```python
from build123d import *

# Parameters (mm, degrees)
SKETCH1_R               = 6.985
BOSS_EXTRUDE1_DEPTH     = 2.54
BOSS_EXTRUDE2_DEPTH     = 81.28
BOSS_EXTRUDE3_DEPTH     = 2.54
FILLET1_R               = 2.54
SKETCH4_R               = 7.62
BOSS_EXTRUDE4_DEPTH     = 12.7
CUT_EXTRUDE1_DEPTH      = 101.243554531
CUT_EXTRUDE1_DEPTH_BACK = 101.243554531
SKETCH5_R               = 1.905


with BuildPart() as part:
    # Sketch1 → Boss-Extrude1 (new body)
    with BuildSketch(Plane.XY):
        Circle(SKETCH1_R)
    extrude(amount=BOSS_EXTRUDE1_DEPTH)

    # Sketch2 → Boss-Extrude2 (add)
    with BuildSketch(Plane.XY.offset(2.54)):
        Polygon((-0.635, -0.635), (-5.715, -0.635), (-5.715, 0.635), (-0.635, 0.635), (-0.635, 5.715), (0.635, 5.715), (0.635, 0.635), (5.715, 0.635), (5.715, -0.635), (0.635, -0.635), (0.635, -5.715), (-0.635, -5.715), align=None)
    extrude(amount=BOSS_EXTRUDE2_DEPTH)

    # Sketch3 → Boss-Extrude3 (add)
    with BuildSketch(Plane.XY.offset(83.82)):
        Polygon((-3.175, 0.635), (-0.635, 0.635), (-0.635, 3.175), (0.635, 3.175), (0.635, 0.635), (3.175, 0.635), (3.175, -0.635), (0.635, -0.635), (0.635, -3.175), (-0.635, -3.175), (-0.635, -0.635), (-3.175, -0.635), align=None)
    extrude(amount=BOSS_EXTRUDE3_DEPTH)

    # Fillet1
    fillet1_edges = [part.edges().sort_by_distance(p)[0] for p in [
        (0, -3.175, 83.82),
        (3.175, 0, 83.82),
        (0, 3.175, 83.82),
        (-3.175, 0, 83.82),
    ]]
    fillet(fillet1_edges, radius=FILLET1_R - 0.0001)  # a hair under: the kernel refuses the full size

    # Sketch4 → Boss-Extrude4 (add)
    with BuildSketch(Plane.XY.offset(86.36)):
        Circle(SKETCH4_R)
    extrude(amount=BOSS_EXTRUDE4_DEPTH)

    # Sketch5 → Cut-Extrude1 (cut, two sides: drawn at the far end of the back side and taken through both)
    with BuildSketch(Plane(origin=(5.715, 0, 0), x_dir=(0, 0, -1), z_dir=(1, 0, 0)).offset(-CUT_EXTRUDE1_DEPTH_BACK)):
        with Locations(Location((-92.458470984, 0, 0), (0, 0, 180.000000004))):
            Circle(SKETCH5_R)
    extrude(amount=CUT_EXTRUDE1_DEPTH + CUT_EXTRUDE1_DEPTH_BACK, mode=Mode.SUBTRACT)


solid = part.part
```
Can you work these out from the model? Positions are in its coordinate system, mm. A direction names the side the tool comes from. Round coordinates to 2 decimals unless told otherwise and drop trailing zeros. Loops run counter-clockwise (first coordinate to the right, second up) from the corner with the lowest first, then second, coordinate; pieces in that order, holes last.
Item 1: Which directions (+Z, -Z, +X, -X, +Y, -Y) give clear straight access to the entire face, cutting with the end or side of a thin tool? Please do faces 4 (the cylindrical face through (-3.939, 0.009, 84.544)), 5 (the cylindrical face through (3.939, -0.009, 84.544)), 6 (the flat face through (-3, 0.635, 44)), 7 (the flat face through (3, -0.635, 44)), 8 (the flat face through (2, -2, 86.36)).
Item 2: Suppose I cut it at A-A, the plane z = 78.5. Write out the boundary of the cut face in (x, y) (3 decimals).
Item 3: Suppose I cut it at B-B, the plane x = 1.5. Write out the boundary of the cut face in (y, z) (3 decimals), then the cut area to 3 significant figures.
Item 4: Will these pins go through, and if not, where does the flat tip stop? pin 1 Ø2 at (y, z) = (0.5, 28.5) entering from -X (3 decimals); pin 2 Ø1.5 at (y, z) = (2, 28) entering from +X (3 decimals); pin 3 Ø2 at (x, z) = (-0.5, 29) entering from +Y (3 decimals); pin 4 Ø5 at (x, y) = (5.5, -5.5) entering from -Z.
Item 5: If we mould it in two halves opening along Y, with no side actions, what happens to faces 1 (the flat face through (3, 0.635, 44)), 2 (the flat face through (0.635, -3, 44)), 3 (the cylindrical face through (-0.107, -0.572, 94.276))? For each: +Y half, -Y half, draft (parallel to the pull), parting line (faces both ways), or undercut.
Item 6: Please list where these lines run through material, in increasing order: L1, parallel to Z at x = 3, y = 3; L2, parallel to Z at x = -4, y = 0; L3, parallel to Z at x = 6, y = 0.5.
Reported:
1. face 4: -X, +Y, -Y
1. face 5: +X, +Y, -Y
1. face 6: -X, +Y
1. face 7: +X, -Y
1. face 8: none
2. outline: (-5.715, -0.635) - (-0.635, -0.635) - (-0.635, -5.715) - (0.635, -5.715) - (0.635, -0.635) - (5.715, -0.635) - (5.715, 0.635) - (0.635, 0.635) - (0.635, 5.715) - (-0.635, 5.715) - (-0.635, 0.635) - (-5.715, 0.635) - close
3. outline: (-7.471, 86.36) - (-0.635, 86.36) - (-0.635, 2.54) - (-6.822, 2.54) - (-6.822, 0) - (6.822, 0) - (6.822, 2.54) - (0.635, 2.54) - (0.635, 86.36) - (7.471, 86.36) - (7.471, 99.06) - (-7.471, 99.06) - close; hole circle Ø3.81 at (0, 92.458)
3. area: 319 mm2
4. pin 1: stops at x = -5.715
4. pin 2: stops at x = 0.635
4. pin 3: stops at y = 5.715
4. pin 4: stops at z = 0
5. face 1: +Y half
5. face 2: draft
5. face 3: undercut
6. L1: z = 0 to 2.54, 86.36 to 99.06
6. L2: z = 0 to 84.49, 86.36 to 90.55, 94.36 to 99.06
6. L3: z = 0 to 2.54, 86.36 to 90.62, 94.3 to 99.06
